Autodesk Inventor part; units mm, degrees
ref_plane "YZ Plane" through (0, 0, 0) normal (1, 0, 0) x (0, 1, 0)
ref_plane "XZ Plane" through (0, 0, 0) normal (0, 1, 0) x (-1, 0, 0)
sketch "Sketch1" plane through (0, 0, 0) normal (0, 0, 1) x (1, 0, 0)
  line L0 (0, 3.937) -> (0, 34.925)
  line L1 (0, 34.925) -> (3.175, 34.925)
  line L2 (3.175, 34.925) -> (3.175, 3.175)
  line L3 (3.175, 3.175) -> (81.407, 3.175)
  line L4 (81.407, 3.175) -> (81.407, 53.975)
  line L5 (81.407, 53.975) -> (84.582, 53.975)
  line L6 (84.582, 53.975) -> (84.582, 3.937)
  line L7 (80.645, 0) -> (3.937, 0)
  arc A0 (80.645, 0) -> (84.582, 3.937) centre (80.645, 3.937) ccw
  arc A1 (0, 3.937) -> (3.937, 0) centre (3.937, 3.937) ccw
  point P0 (0, 0)
  dimension "d0" = 34.925
  dimension "d1" = 3.175
  dimension "d2" = 31.75
  dimension "d3" = 78.232
  dimension "d4" = 50.8
  dimension "d5" = 3.175
  dimension "d6" = 3.937
  dimension "d7" = 3.937
extrude "Extrusion1" add sketch "Sketch1" along normal mid plane 203.2
sketch "Sketch2" plane through (84.582, 3.937, 101.6) normal (1, 0, 0) x (0, 0, -1)
  line L0 (203.2, -0.762) -> (0, -0.762)
  line L1 (203.2, 50.038) -> (0, 50.038)
  line L2 (73.025, -0.762) -> (38.1, -0.762)
  line L3 (38.1, -0.762) -> (38.1, 50.038)
  line L4 (38.1, 50.038) -> (73.025, 50.038)
  line L5 (73.025, 50.038) -> (73.025, -0.762)
  line L6 (0, 0) -> (0, 50.038)
  point P0 (101.6, -3.937)
  point P1 (38.1, -0.762)
  dimension "d10" = 38.1
  dimension "d11" = 34.925
extrude "Extrusion2" cut sketch "Sketch2" against normal through all
properties part number "2020 Front Plate"
Work out the finished part from the listing and answer in its coordinate system (mm). A direction names the side the tool comes from. Give positions to 0.01 mm unless a question says otherwise; leave off trailing zeros. Write each loop counter-clockwise with the first axis right and the second up, starting at its lowest first coordinate (ties: lowest second). Pieces come first, ordered by that corner, then holes. Notation, with made-up numbers: (-14.75, 44) - (41.25, 44) arc R23 cw to (41.25, 76) - close; hole circle Ø1 at (54, -0.75). An arc over 180 degrees is marked (long way). One line per item, written item: value. Start each with the question number.
1. Given pin 1 (8 mm diameter, centred on y = 41.5, z = -75.5, fed in from -X); pin 2 (1.6 mm diameter, centred on x = 1.5, z = 88, fed in from +Y) (3 decimals); pin 3 (1 mm diameter, centred on x = 62.5, z = -81, fed in from +Y) (3 decimals), each flat-ended and moving along its own axis, determine where each tip first touches the part or whether it passes through.
2. Find section D-D (x = 47.5). Write down the section's boundary in (y, z) (3 decimals), then the cut area to 3 significant figures.
3. Consider probe 1 along X at (y, z) = (13.5, 78.5) (3 decimals); probe 2 along Y at (x, z) = (69, -75) (3 decimals); probe 3 along X at (y, z) = (35.5, -63.5). Determine where each line is inside the solid, lowest interval first.
4. Find section C-C (z = -32.5). Write down the section's boundary in (x, y) (3 decimals).
5. For faces 1 (the flat face through (81.407, 28, -37)), 2 (the flat face through (43, 0, -1)), determine the directions among +Z, -Z, +X, -X, +Y, -Y from which every point of the face is accessible in a straight line to the end or side of a thin tool.
6. Find section B-B (y = 17). Write down the section's boundary in (x, z) (3 decimals).
7. Find section A-A (y = 37). Write down the section's boundary in (x, z) (3 decimals), then the cut area to 3 significant figures.
8. For a pull along X with two mould halves and no side action, classify faces 3 (the flat face through (3.175, 19, -37)), 4 (the flat face through (84.582, 29, 82)), 5 (the flat face through (0, 19, -37)) as +X half, -X half, draft (parallel to the pull), parting line (faces both ways), or undercut.
Geometry results:
1. pin 1: x = 81.41
1. pin 2: y = 34.925
1. pin 3: y = 3.175
2. outline: (0, -101.6) - (3.175, -101.6) - (3.175, 101.6) - (0, 101.6) - close
2. area: 645 mm2
3. probe 1: 0 to 3.175, 81.407 to 84.582
3. probe 2: 0 to 3.175
3. probe 3: 81.41 to 84.58
4. outline: (0, 3.937) arc R3.937 ccw to (3.937, 0) - (80.645, 0) arc R3.937 ccw to (84.582, 3.937) - (84.582, 53.975) - (81.407, 53.975) - (81.407, 3.175) - (3.175, 3.175) - (3.175, 34.925) - (0, 34.925) - close
5. face 1: +Z, -Z, +Y
5. face 2: +Z, -Z, +X, -X, -Y
6. outline: (0, -101.6) - (3.175, -101.6) - (3.175, 28.575) - (0, 28.575) - close; (0, 63.5) - (3.175, 63.5) - (3.175, 101.6) - (0, 101.6) - close; (81.407, -101.6) - (84.582, -101.6) - (84.582, 28.575) - (81.407, 28.575) - close; (81.407, 63.5) - (84.582, 63.5) - (84.582, 101.6) - (81.407, 101.6) - close
7. outline: (81.407, -101.6) - (84.582, -101.6) - (84.582, 28.575) - (81.407, 28.575) - close; (81.407, 63.5) - (84.582, 63.5) - (84.582, 101.6) - (81.407, 101.6) - close
7. area: 534 mm2
8. face 3: undercut
8. face 4: +X half
8. face 5: -X half
